Verification items for the finished model (mm, model axes). Give positions to 0.01 mm unless a question says otherwise; leave off trailing zeros. Write each loop counter-clockwise with the first axis right and the second up, starting at its lowest first coordinate (ties: lowest second). Pieces come first, ordered by that corner, then holes. Notation, with made-up numbers: M 80.5,24 L 104.5,24 A36 cw 104.5,62 Z; hole C 28,88.5 d2. An arc over 180 degrees is marked long. Answer as a JSON object with one key per item and string values.
```python
from build123d import *


with BuildPart() as part:
    # Sketch1 → Revolve1 (revolve)
    with BuildSketch(Plane.XY, mode=Mode.PRIVATE) as revolve1_sk:
        with BuildLine():
            Line((0.066666667, 4.95), (1.6877501, 4.95))
            ThreePointArc((1.6877501, 4.95), (2, 5), (2.3122499, 4.95))
            Line((2.3122499, 4.95), (3.933333333, 4.95))
            ThreePointArc((3.933333333, 4.95), (3.980473785, 4.969526215), (4, 5.016666667))
            Line((4, 5.016666667), (4, 5.8))
            ThreePointArc((4, 5.8), (3.941421356, 5.941421356), (3.8, 6))
            Line((3.8, 6), (0.2, 6))
            ThreePointArc((0.2, 6), (0.058578644, 5.941421356), (0, 5.8))
            Line((0, 5.8), (0, 5.016666667))
            ThreePointArc((0, 5.016666667), (0.019526215, 4.969526215), (0.066666667, 4.95))
        make_face()
    revolve(revolve1_sk.sketch.rotate(Axis((4, 0, 0), (-1, 0, 0)), 270), axis=Axis((4, 0, 0), (-1, 0, 0)))


solid = part.part
```
1) Thickness scan on L1, parallel to Y at x = 0.85, z = 0; L2, parallel to Y at x = 1.25, z = 4; L3, parallel to Z at x = 1, y = 2. Record the ranges inside material, lowest first.
Completed:
{"L1": "y = -6 to -4.95, 4.95 to 6", "L2": "y = -4.47 to -2.92, 2.92 to 4.47", "L3": "z = -5.66 to -4.53, 4.53 to 5.66"}
2) Go/stop test with flat-tipped pins: pin 1 (1 mm diameter, centred on x = 2.5, z = 4.5, fed in from -Y); pin 2 (1.5 mm diameter, centred on x = 2.5, y = -4, fed in from -Z). Record where each tip stops, or that it passes through.
Completed:
{"pin 1": "stops at y = -4.47", "pin 2": "stops at z = -5.04"}
3) Section check C-C on x = 3.65. Record the boundary of the cut face in (y, z), and give its area (3 significant figures).
Completed:
{"outline": "C 0,0 d12; hole C 0,0 d9.9", "area": "36.1 mm2"}
4) Section check A-A on z = 0. Record the boundary of the cut face in (x, y), and give its area (3 significant figures).
Completed:
{"outline": "M 0,-5.8 A0.2 ccw 0.2,-6 L 3.8,-6 A0.2 ccw 4,-5.8 L 4,-5.02 A0.07 ccw 3.93,-4.95 L 2.31,-4.95 A1 cw 1.69,-4.95 L 0.07,-4.95 A0.07 ccw 0,-5.02 Z; M 0,5.02 A0.07 ccw 0.07,4.95 L 1.69,4.95 A1 cw 2.31,4.95 L 3.93,4.95 A0.07 ccw 4,5.02 L 4,5.8 A0.2 ccw 3.8,6 L 0.2,6 A0.2 ccw 0,5.8 Z", "area": "8.32 mm2"}
5) Release check for a two-part mould opening along Y. For faces 1 (the face through (0.89, 1.49, 4.72)), 2 (the face through (0, 5, -2)), 3 (the face through (1.975, 1.802, 5.723)) record: pulls with the +Y half, pulls with the -Y half, needs draft (parallel to the pull), parting line crosses it, or undercut.
Completed:
{"face 1": "undercut", "face 2": "needs draft", "face 3": "parting line crosses it"}
